Design review of the part built by this model. Coordinates are the model's own, in mm. Give positions to 0.01 mm unless a question says otherwise; leave off trailing zeros. Write each loop counter-clockwise with the first axis right and the second up, starting at its lowest first coordinate (ties: lowest second). Pieces come first, ordered by that corner, then holes.
Solid Edge part; units mm, degrees
sketch "Sketch1" plane through (0, 0, 0) normal (0, 0, 1) x (1, 0, 0)
  circle A0 centre (-68.9258, 50.0648) radius 120
extrude "Protrusion1" add sketch "Sketch1" along normal blind 10
sketch "Sketch2" plane through (-68.9258, 50.0648, 10) normal (0, 0, 1) x (1, 0, 0)
  circle A0 centre (0, 100) radius 5
extrude "Cutout1" cut sketch "Sketch2" against normal through all
pattern_circular "Pattern1" count 10 over 360 about axis through (-68.9258, 50.0648, 10) along (0, 0, -1) of "Cutout1"
sketch "Sketch3" plane through (-68.9258, 50.0648, 10) normal (0, 0, 1) x (1, 0, 0)
  circle A0 centre (0, 0) radius 25
extrude "Cutout2" cut sketch "Sketch3" against normal through all
(1) Consider section C-C, the plane x = -28. Give the boundary of the cut face in (y, z).
Resolved:
outline: (-62.74, 0) - (162.87, 0) - (162.87, 10) - (-62.74, 10) - close
(2) Consider section B-B, the plane y = 58. Give the boundary of the cut face in (x, z), then the cut area to 3 significant figures.
Resolved:
outline: (-188.66, 0) - (-92.63, 0) - (-92.63, 10) - (-188.66, 10) - close; (-45.22, 0) - (50.81, 0) - (50.81, 10) - (-45.22, 10) - close
area: 1,920 mm2
(3) Consider section D-D, the plane y = -42. Give the boundary of the cut face in (x, z).
Resolved:
outline: (-145.89, 0) - (8.04, 0) - (8.04, 10) - (-145.89, 10) - close
(4) Mouldability with a two-part tool opening along X and no side actions: class faces 1 (the face through (-71, 25, 10)), 2 (the face through (-124.729, 134.985, 5.07)), 3 (the face through (-188.81, 44.79, 4.93)) as pulls with the +X half, pulls with the -X half, needs draft (parallel to the pull), parting line crosses it, or undercut.
Resolved:
face 1: needs draft
face 2: undercut
face 3: parting line crosses it
(5) To check wall thickness, follow L1, parallel to X at y = -31, z = 6; L2, parallel to X at y = 59.5, z = 1; L3, parallel to Y at x = -165, z = 5.5. State the ranges of each line that lie inside material, in increasing order.
Resolved:
L1: x = -157.4 to -132.7, -122.71 to -15.14, -5.15 to 19.55
L2: x = -188.55 to -92.08, -45.77 to 50.7
L3: y = -21.84 to 14.26, 24.07 to 76.06, 85.87 to 121.97
(6) Clearance check with flat-ended pins moving along their axes: P1, Ø8, axis at x = -10.15, y = -30.84, coming from the +Z side; P2, Ø4, axis at y = -11, z = 8.5, coming from the +X side; P3, Ø6, axis at x = -11.5, z = 8.5, coming from the -Y side; P4, Ø2, axis at x = -14.5, z = 6, coming from the +Y side. State where each tip first meets the part, or that it passes through.
Resolved:
P1: passes through
P2: stops at x = 35.53
P3: stops at y = -56.88
P4: stops at y = 157.52
